```python
from build123d import *

# Parameters (mm, degrees)
SUSP_RL_UCA_BALL_JOINT_PROFILE_R  = 17
SUSP_RL_LCA_BALL_JOINT_PROFILE_R  = 17
SUSP_RL_UPRIGHT_KINGPIN_START     = -15.170463608
SUSP_RL_UPRIGHT_KINGPIN_OUTLINE_R = 17
SUSP_RL_UPRIGHT_KINGPIN_DEPTH     = 237.229999131
SUSP_RL_UPRIGHT_SPINDLE_PROFILE_R = 20
SUSP_RL_UPRIGHT_ARM_PROFILE_R     = 9
SUSP_RL_HUB_PROFILE_R             = 55


# Read off the part's stored shape, not the designer's step: SUSP_RL_upright_kingpin
with BuildPart() as part:
    # SUSP_RL_UCA_ball_joint: sweep along a curve in space
    with BuildLine() as susp_rl_uca_ball_joint_path:
        Line((-521.613651, 1419.6, -302.481439), (-517.770606, 1419.6, -328.195852))
    # SUSP_RL_UCA_ball_joint profile (on start of the path) → SUSP_RL_UCA_ball_joint (sweep)
    with BuildSketch(Plane(origin=(-521.613651, 1419.6, -302.481439), x_dir=(-0.9890158620797268, 0, -0.14780941970894487), z_dir=(0.14780941970894487, 0, -0.9890158620797268))):
        Circle(SUSP_RL_UCA_BALL_JOINT_PROFILE_R)
    sweep(path=susp_rl_uca_ball_joint_path.line)


with BuildPart() as body_2:
    # SUSP_RL_LCA_ball_joint: sweep along a curve in space
    with BuildLine() as susp_rl_lca_ball_joint_path:
        Line((-560.521522, 1419.6, -42.1427938), (-556.678478, 1419.6, -67.8572062))
    # SUSP_RL_LCA_ball_joint profile (on start of the path) → SUSP_RL_LCA_ball_joint (sweep)
    with BuildSketch(Plane(origin=(-560.521522, 1419.6, -42.1427938), x_dir=(-0.9890158671980833, 0, -0.14780938546121916), z_dir=(0.14780938546121916, 0, -0.9890158671980833))):
        Circle(SUSP_RL_LCA_BALL_JOINT_PROFILE_R)
    sweep(path=susp_rl_lca_ball_joint_path.line)


with BuildPart() as susp_rl_upright_kingpin_tool:
    # SUSP_RL_upright_kingpin outline → SUSP_RL_upright_kingpin (new body)
    with BuildSketch(Plane(origin=(0, 0, 0), x_dir=(0.9890158635477251, 0, 0.14780940988633906), z_dir=(0.14780940988633903, 0, -0.9890158635477251)).offset(SUSP_RL_UPRIGHT_KINGPIN_START)):
        with Locations((-560.593778922, -1419.6)):
            Circle(SUSP_RL_UPRIGHT_KINGPIN_OUTLINE_R)
    extrude(amount=SUSP_RL_UPRIGHT_KINGPIN_DEPTH)


with BuildPart() as part_1:
    add(part.part)


with BuildPart() as part_2:
    # SUSP_RL_upright_kingpin: joined with susp_rl_upright_kingpin_tool
    add(part_1.part.fuse(susp_rl_upright_kingpin_tool.part, body_2.part, tol=0.00001))

    # SUSP_RL_upright_spindle: sweep along a curve in space
    with BuildLine() as susp_rl_upright_spindle_path:
        Line((-542.552954, 1419.6, -162.373292), (-593.584449, 1419.6, -170))
    # SUSP_RL_upright_spindle profile (on start of the path) → SUSP_RL_upright_spindle (sweep)
    with BuildSketch(Plane(origin=(-542.552954, 1419.6, -162.373292), x_dir=(0.14780941059704947, 0, -0.9890158634415087), z_dir=(-0.9890158634415087, 0, -0.14780941059704947))):
        Circle(SUSP_RL_UPRIGHT_SPINDLE_PROFILE_R)
    sweep(path=susp_rl_upright_spindle_path.line)

    # SUSP_RL_upright_arm: sweep along a curve in space
    with BuildLine() as susp_rl_upright_arm_path:
        Line((-549.94905, 1419.6, -112.88486), (-520.81, 1474.2, -108.53))
    # SUSP_RL_upright_arm profile (on start of the path) → SUSP_RL_upright_arm (sweep)
    with BuildSketch(Plane(origin=(-549.94905, 1419.6, -112.88486), x_dir=(0.8822250985406449, -0.47082786186137016, 0), z_dir=(0.46966656036901244, 0.8800490817699289, 0.07019213450982756))):
        Circle(SUSP_RL_UPRIGHT_ARM_PROFILE_R)
    sweep(path=susp_rl_upright_arm_path.line)

    # SUSP_RL_hub: sweep along a curve in space
    with BuildLine() as susp_rl_hub_path:
        Line((-573.591303, 1419.6, -169.476461), (-613.577596, 1419.6, -170.523539))
    # SUSP_RL_hub profile (on start of the path) → SUSP_RL_hub (sweep)
    with BuildSketch(Plane(origin=(-573.591303, 1419.6, -169.476461), x_dir=(0.026176949998200902, 0, -0.9996573249312944), z_dir=(-0.9996573249312944, 0, -0.026176949998200902))):
        Circle(SUSP_RL_HUB_PROFILE_R)
    sweep(path=susp_rl_hub_path.line)


solid = part_2.part
```
Model file for the job. Use its own axes, mm. A direction names the side the tool comes from. Give positions to 0.01 mm unless a question says otherwise; leave off trailing zeros. Loops run counter-clockwise (first coordinate to the right, second up) from the corner with the lowest first, then second, coordinate; pieces in that order, holes last. Notation, with made-up numbers: (-30.5, 37.5) - (-16.5, 37.5) arc R21 cw to (-16.5, 55.5) - close; hole circle Ø1 at (-5.5, -21). An arc over 180 degrees is marked (long way). One line per item, written item: value. Start each with the question number.
1. Probe L1, parallel to X at y = 1423, z = -137; L2, parallel to X at y = 1381.5, z = -132; L3, parallel to Y at x = -534, z = -270. List the from-to ranges inside material, lowest first. Write a range as from..to.
2. Which spindle directions (+Z, -Z, +X, -X, +Y, -Y) get a long thin tool onto all of the face, cutting with end or side? Do faces 1 (the flat face through (-560.29, 1419.84, -42.11)), 2 (the cylindrical face through (-594.176, 1473.292, -158.088)). Say none if no direction does.
3. Slice it at A-A (y = 1381.5). List the corners of the cut face in (x, z), plus the area to 3 significant figures.
4. Pin check, flat tips, straight feed: pin 1 (4 mm diameter, centred on x = -529, z = -265, fed in from +Y); pin 2 (6 mm diameter, centred on y = 1411, z = -294, fed in from +X); pin 3 (5 mm diameter, centred on x = -562.5, y = 1440.5, fed in from +Z). Stop position of each tip, or through.
Solution:
1. L1: x = -614.46..-574.44, -563.19..-529.5
1. L2: x = -614.59..-574.57
1. L3: y = 1404.32..1434.88
2. face 1: +Z, -X, +Y, -Y
2. face 2: none
3. outline: (-614.62, -130.87) - (-612.54, -210.18) - (-572.55, -209.13) - (-574.63, -129.82) - close
3. area: 3,170 mm^2
4. pin 1: stops at y = 1436.6
4. pin 2: stops at x = -506.56
4. pin 3: stops at z = -157.42
